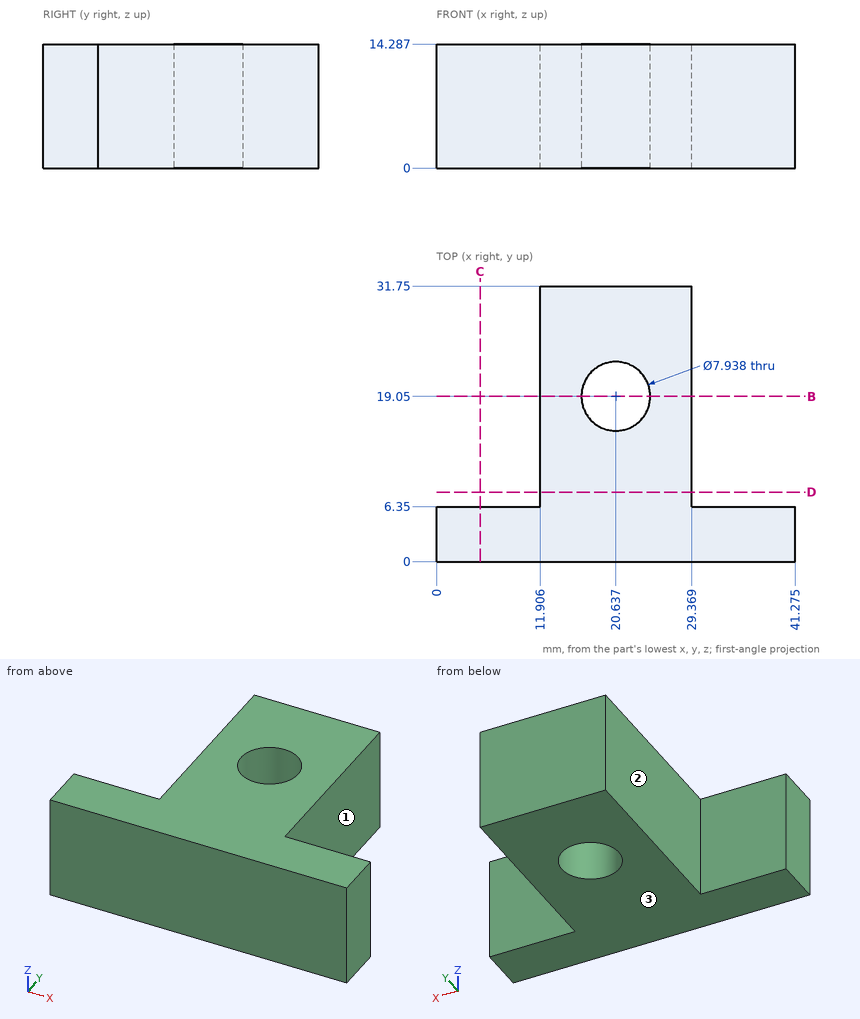
For this review, use the dimensioned drawing (mm, ordinates from the lowest corner) and the shaded views. A direction names the side the tool comes from. Coordinates: 2 decimals unless noted, no trailing zeros. Order: outer loops, then holes, each group sorted by start corner. A loop starts at its lowest first (then second) coordinate and runs counter-clockwise, first axis right, second up. Notation, with made-up numbers: (47.5, 34.25) - (51.5, 34.25) arc R11 cw to (51.5, 54.25) - close; hole circle Ø2 at (41, 67.25). An arc over 180 degrees is marked (long way). Answer as a JSON object with one key per item and string values. Group by question number.
1. We need section B-B on y = 19.05. State the section outline as (x, z) points, then the cut area to 3 significant figures.
2. For probe 1 along Y at (x, z) = (9, 13); probe 2 along X at (y, z) = (13, 10.75); probe 3 along Y at (x, z) = (23, 7.5), list the stretches that pass through material, from the lowest coordinate up.
3. We need section D-D on y = 8. State the section outline as (x, z) points.
4. For the marked faces 1, 2 and 3, list the 3-axis set-ups (+Z, -Z, +X, -X, +Y, -Y) from which the entire face can be reached by the end or side of a thin tool; tool diameter is ignored.
5. Clearance check with flat-ended pins moving along their axes: P1, Ø6, axis at y = 10.5, z = 4, coming from the -X side; P2, Ø6, axis at x = 35.5, z = 9.5, coming from the +Y side; P3, Ø1, axis at y = 25.5, z = 5.5, coming from the +X side. State where each tip first meets the part, or that it passes through.
6. We need section C-C on x = 5. State the section outline as (y, z) points.
Final values:
{
 "1": {"outline": "(11.91, 0) - (16.67, 0) - (16.67, 14.29) - (11.91, 14.29) - close; (24.61, 0) - (29.37, 0) - (29.37, 14.29) - (24.61, 14.29) - close", "area": "136 mm²"},
 "2": {"probe 1": "0 to 6.35", "probe 2": "11.91 to 29.37", "probe 3": "0 to 15.86, 22.24 to 31.75"},
 "3": {"outline": "(11.91, 0) - (29.37, 0) - (29.37, 14.29) - (11.91, 14.29) - close"},
 "4": {"face 1": "+Z, -Z, +X, +Y", "face 2": "+Z, -Z, -X, +Y", "face 3": "-Z, +X, -X, +Y, -Y"},
 "5": {"P1": "x = 11.91", "P2": "y = 6.35", "P3": "x = 29.37"},
 "6": {"outline": "(0, 0) - (6.35, 0) - (6.35, 14.29) - (0, 14.29) - close"}
}
